from build123d import *

# Parameters (mm, degrees)
SKETCH1_R           = 1
BOSS_EXTRUDE1_DEPTH = 4.8
FILLET1_R           = 0.5


with BuildPart() as part:
    # Sketch1 → Boss-Extrude1 (new body)
    with BuildSketch(Plane(origin=(0, 0, 0), x_dir=(1, 0, 0), z_dir=(0, 1, 0))):
        with BuildLine():
            Line((0, 0), (0, 10.109966322))
            Line((0, 10.109966322), (4.6, 10.109966322))
            Line((4.6, 10.109966322), (4.6, 1.714229872))
            Line((4.6, 1.714229872), (27.967443814, 1.714229872))
            Line((27.967443814, 1.714229872), (27.967443814, 14.126132931))
            Line((27.967443814, 14.126132931), (32.567443814, 14.126132931))
            Line((32.567443814, 14.126132931), (32.567443814, 1.22414249))
            ThreePointArc((32.567443814, 1.22414249), (31.144234193, -1.974320184), (27.900175322, -3.290287941))
            Line((27.900175322, -3.290287941), (17.770133396, -3.290287941))
            ThreePointArc((17.770133396, -3.290287941), (16.223398412, -2.475294407), (14.868870839, -3.580671549))
            Line((14.868870839, -3.580671549), (10.12183502, -3.580671549))
            ThreePointArc((10.12183502, -3.580671549), (7.826617972, -1.836209825), (5.897335796, -3.978413896))
            ThreePointArc((5.897335796, -3.978413896), (2.124711402, -3.210585182), (0, 0))
        make_face()
        with Locations((28.067931627, -0.839685826)):
            Circle(SKETCH1_R, mode=Mode.SUBTRACT)
        with Locations((30.267443814, 8.215801601)):
            Circle(SKETCH1_R, mode=Mode.SUBTRACT)
        with Locations((2.212966765, 8.215801601)):
            Circle(SKETCH1_R, mode=Mode.SUBTRACT)
        with Locations((13.539270752, -0.839685826)):
            Circle(SKETCH1_R, mode=Mode.SUBTRACT)
    extrude(amount=BOSS_EXTRUDE1_DEPTH)

    # Fillet1
    fillet1_edges = [part.edges().sort_by_distance(p)[0] for p in [
        (27.967443814, 2.4, -14.126132931),
        (32.567443814, 2.4, -14.126132931),
        (0, 2.4, -10.109966322),
        (4.6, 2.4, -10.109966322),
    ]]
    fillet(fillet1_edges, radius=FILLET1_R)


solid = part.part
Geometry: final body of the model. Coordinates: model frame, mm. A direction names the side the tool comes from. Round coordinates to 2 decimals unless told otherwise and drop trailing zeros. Loops run counter-clockwise (first coordinate to the right, second up) from the corner with the lowest first, then second, coordinate; pieces in that order, holes last. Notation, with made-up numbers: (-9.5, -38) - (35.5, -38) arc R18 ccw to (35.5, -16) - close; hole circle Ø1 at (-38.75, 1). An arc over 180 degrees is marked (long way). Write each question's results on one line, items separated by ' | '. Start each with the question number.
1) Cut plane D-D on x = 20.5. Return loops of the section in (y, z), then the cut area to 3 significant figures.
2) Cut plane B-B on x = 13.5. Return loops of the section in (y, z).
3) Mould query, pull axis Z, two halves, no side actions, for faces 5 (the face through (0, 2, -5)), 6 (the face through (29.27, 2.37, -8.26)), 7 (the face through (16, 2, -1.714)). Classes: released by +Z, released by -Z, zero draft, split by the parting line, or undercut.
4) Cut plane A-A on z = -3.25. Return loops of the section in (x, y), then the cut area to 3 significant figures.
5) Cut plane C-C on y = 2.9. Return loops of the section in (x, z).
6) Access query for faces 1 (the face through (23, 2, 3.29)), 2 (the face through (27.967, 2, -8)), 3 (the face through (2, 2, -10.11)), 4 (the face through (17, 4.8, -1)). Directions: +Z, -Z, +X, -X, +Y, -Y. A direction counts if a zero-diameter tool reaches every point of the face in a straight line with its end or side. Return the directions, or none.
7) Line query: probe 1 along X at (y, z) = (1.35, -4.25); probe 2 along X at (y, z) = (2.3, 0); probe 3 along X at (y, z) = (3.35, -13). Output: solid intervals per line, ascending. Write a range as [from, to].
8) First-contact query: P1, Ø1, axis at x = 26, y = 3, coming from the +Z side; P2, Ø1.6, axis at x = 13.54, z = 0.84, coming from the -Y side; P3, Ø2.5, axis at x = 12.5, y = 3.5, coming from the -Z side; P4, Ø2.5, axis at x = 12, y = 3, coming from the +Z side. Flat tips, straight axial feed; report the tip coordinate or a pass-through.
Verdict:
1) outline: (0, -1.71) - (4.8, -1.71) - (4.8, 3.29) - (0, 3.29) - close | area: 24.0 mm2
2) outline: (0, -1.71) - (4.8, -1.71) - (4.8, -0.16) - (0, -0.16) - close; (0, 1.84) - (4.8, 1.84) - (4.8, 3.58) - (0, 3.58) - close
3) face 5: zero draft | face 6: undercut | face 7: released by -Z
4) outline: (0, 0) - (4.6, 0) - (4.6, 4.8) - (0, 4.8) - close; (27.97, 0) - (32.57, 0) - (32.57, 4.8) - (27.97, 4.8) - close | area: 44.2 mm2
5) outline: (0, -9.61) arc R0.5 ccw to (0.5, -10.11) - (4.1, -10.11) arc R0.5 ccw to (4.6, -9.61) - (4.6, -1.71) - (27.97, -1.71) - (27.97, -13.63) arc R0.5 ccw to (28.47, -14.13) - (32.07, -14.13) arc R0.5 ccw to (32.57, -13.63) - (32.57, -1.22) arc R4.68 ccw to (27.9, 3.29) - (17.77, 3.29) arc R1.58 cw to (14.87, 3.58) - (10.12, 3.58) arc R2.13 cw to (5.9, 3.98) arc R5.03 ccw to (0, 0) - close; hole circle Ø2 at (2.21, -8.22); hole circle Ø2 at (13.54, 0.84); hole circle Ø2 at (28.07, 0.84); hole circle Ø2 at (30.27, -8.22)
6) face 1: +Z, +X, +Y, -Y | face 2: -Z, +Y, -Y | face 3: -Z, -X, +Y, -Y | face 4: +Z, -Z, +X, -X, +Y
7) probe 1: x = [0, 4.6], [27.97, 32.57] | probe 2: x = [0, 13], [14.08, 27.52], [28.61, 32.36] | probe 3: x = [27.97, 32.57]
8) P1: stops at z = 3.29 | P2: passes through | P3: stops at z = -1.71 | P4: stops at z = 3.58
